Here's how the part is built. I have some questions about the finished solid (model axes, mm). A direction names the side the tool comes from. Round coordinates to 2 decimals unless told otherwise and drop trailing zeros. Order: outer loops, then holes, each group sorted by start corner. A loop starts at its lowest first (then second) coordinate and runs counter-clockwise, first axis right, second up.
Autodesk Inventor part; units mm, degrees
ref_plane "YZ Plane" through (0, 0, 0) normal (1, 0, 0) x (0, 1, 0)
ref_plane "XZ Plane" through (0, 0, 0) normal (0, 1, 0) x (-1, 0, 0)
ref_plane "XY Plane" through (0, 0, 0) normal (0, 0, 1) x (1, 0, 0)
sketch "草图1" plane through (0, 0, 0) normal (0, 0, 1) x (1, 0, 0)
  circle A0 centre (0, 0) radius 2.5
  dimension "d0" = 5
extrude "拉伸1" add sketch "草图1" along normal blind 44
sketch "草图2" plane through (0, 0, 0) normal (0, 0, -1) x (-1, 0, 0)
  circle A0 centre (0, 0) radius 5
  dimension "d3" = 10
extrude "拉伸2" add sketch "草图2" along normal blind 2
sketch "草图3" plane through (0, 0, -2) normal (0, 0, -1) x (-1, 0, 0)
  circle A0 centre (0, 0) radius 2.5
  line L0 (2.5, 0) -> (1.25, -2.1651)
  line L1 (1.25, -2.1651) -> (-1.25, -2.1651)
  line L2 (-1.25, -2.1651) -> (-2.5, 0)
  line L3 (-2.5, 0) -> (-1.25, 2.1651)
  line L4 (-1.25, 2.1651) -> (1.25, 2.1651)
  line L5 (1.25, 2.1651) -> (2.5, 0)
  dimension "d6" = 4.3301
extrude "拉伸3" cut sketch "草图3" against normal blind 2 contours L0 L1 L2 L3 L4 L5
thread "螺纹1"
properties part number "Hex Screws used in Desk"
1. If we section it at A-A, the plane x = 0: Write out the boundary of the cut face in (y, z).
Evaluation:
outline: (-5, -2) - (-2.17, -2) - (-2.17, 0) - (2.17, 0) - (2.17, -2) - (5, -2) - (5, 0) - (2.5, 0) - (2.5, 44) - (-2.5, 44) - (-2.5, 0) - (-5, 0) - close
2. I'm going to push flat-ended pins straight in: P1, Ø1.5, axis at y = 0.5, z = 35.5, coming from the -X side; P2, Ø4, axis at y = -1.5, z = 34.5, coming from the +X side; P3, Ø2, axis at x = 0.5, z = 33, coming from the +Y side. Where does each tip first touch, or does it pass through?
Evaluation:
P1: stops at x = -2.5
P2: stops at x = 2.5
P3: stops at y = 2.5
3. If we section it at C-C, the plane z = 6: Write out the boundary of the cut face in (x, y), and give its area (3 significant figures).
Evaluation:
outline: circle Ø5 at (0, 0)
area: 19.6 mm2
4. On a 3-axis mill with a long thin cutter (end or side, diameter ignored), from which of +Z, -Z, +X, -X, +Y, -Y can I reach the whole of each face in a straight line? I mean faces 4 (the flat face through (-2.2, -1, -2)), 5 (the flat face through (0, 2.165, -1)), 6 (the cylindrical face through (-0.54, 2.44, 21.69)). Say none if no direction works.
Evaluation:
face 4: -Z, +X, -X, +Y, -Y
face 5: -Z
face 6: +Z
5. If we mould it in two halves opening along Y, with no side actions, what happens to faces 1 (the flat face through (-2, -2, 0)), 2 (the flat face through (0, -2.165, -1)), 3 (the cylindrical face through (1.08, 4.88, -0.99))? For each: released by +Y, released by -Y, zero draft, split by the parting line, or undercut.
Evaluation:
face 1: zero draft
face 2: undercut
face 3: split by the parting line
6. If we section it at B-B, the plane y = 1.5: Write out the boundary of the cut face in (x, z), and give its area (3 significant figures).
Evaluation:
outline: (-4.77, -2) - (-1.63, -2) - (-1.63, 0) - (1.63, 0) - (1.63, -2) - (4.77, -2) - (4.77, 0) - (2, 0) - (2, 44) - (-2, 44) - (-2, 0) - (-4.77, 0) - close
area: 189 mm2
7. I need wall thicknesses on probe 1 along Z at (x, y) = (3.25, 1.75); probe 2 along Y at (x, z) = (-1.25, 8.5); probe 3 along Z at (x, y) = (1, -1.5). Which ranges of each line are inside material? Lowest first, please.
Evaluation:
probe 1: z = -2 to 0
probe 2: y = -2.17 to 2.17
probe 3: z = 0 to 44
8. If we section it at D-D, the plane y = -3: Write out the boundary of the cut face in (x, z).
Evaluation:
outline: (-4, -2) - (4, -2) - (4, 0) - (-4, 0) - close
